For this review, use the dimensioned drawing (mm, ordinates from the lowest corner) and the shaded views. A direction names the side the tool comes from. Give positions to 0.01 mm unless a question says otherwise; leave off trailing zeros. Write each loop counter-clockwise with the first axis right and the second up, starting at its lowest first coordinate (ties: lowest second). Pieces come first, ordered by that corner, then holes. Notation, with made-up numbers: (44.25, 49.5) - (54.25, 49.5) arc R14 ccw to (54.25, 70.5) - close; hole circle Ø9 at (-13.75, 62.5). An arc over 180 degrees is marked (long way). One line per question, with ' | ' between items. Start each with the question number.
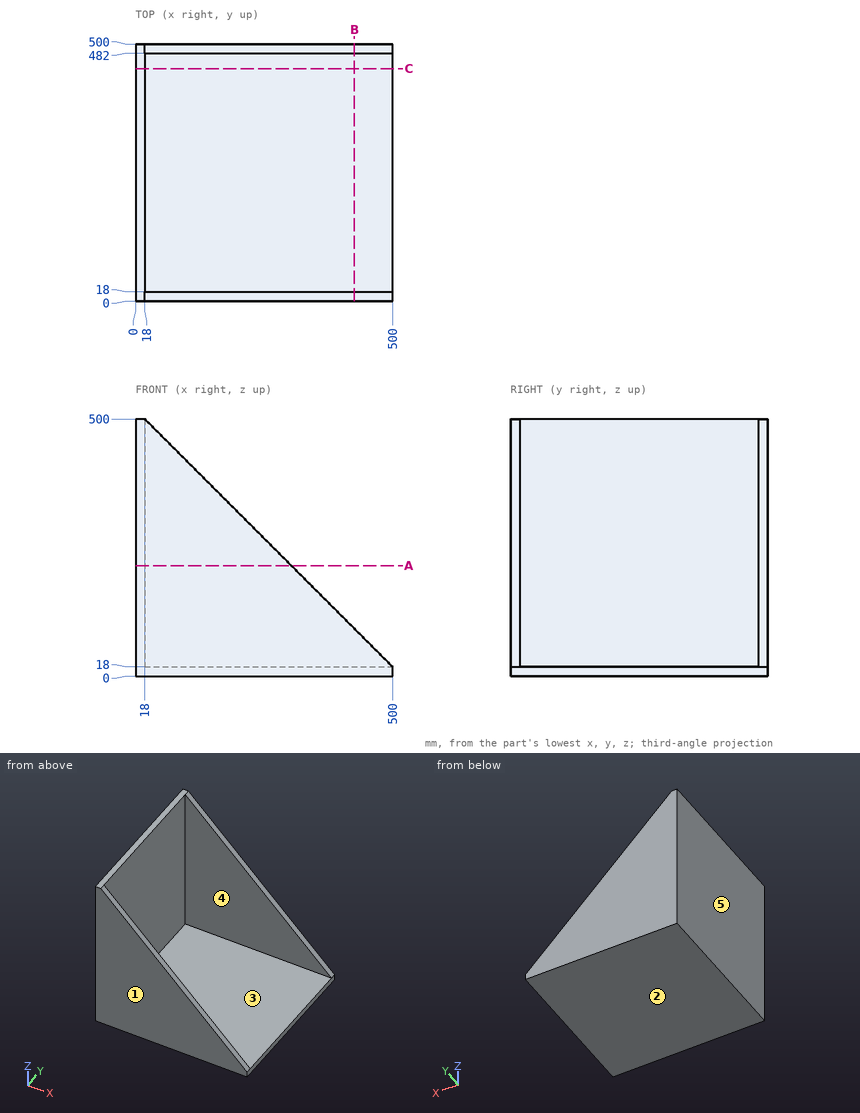
Item 1: Clearance check with a flat-ended pin moving along its axis: P1, Ø3, axis at x = 77.5, y = 74, coming from the +Z side. State where the tip first meets the part, or that it passes through.
Item 2: For probe 1 along Y at (x, z) = (302, 68); probe 2 along X at (y, z) = (246, 169.5), list the stretches that pass through material, from the lowest coordinate up.
Item 3: Machinability: for the marked faces 4 and 5, which of the approach directions +Z, -Z, +X, -X, +Y, -Y give a long, thin tool a straight path to every point of the face, cutting with its end or side? Answer none if there is none.
Item 4: Take a section at A-A (z = 214.5). Give the boundary of the cut face in (x, y), plus the area to 3 significant figures.
Item 5: Take a section at B-B (x = 426). Give the boundary of the cut face in (y, z), plus the area to 3 significant figures.
Item 6: The part is to be moulded in two halves that separate along Y. For the marked faces 1, 2 and 3, say which applies: +Y half, -Y half, draft (parallel to the pull), parting line (faces both ways), or undercut.
Item 7: Take a section at C-C (y = 452). Give the boundary of the cut face in (x, z).
Check sheet entries:
1) P1: stops at z = 18
2) probe 1: y = 0 to 18, 482 to 500 | probe 2: x = 0 to 18
3) face 4: +Z, +X | face 5: +Z, -Z, -X, +Y, -Y
4) outline: (0, 0) - (303.5, 0) - (303.5, 18) - (18, 18) - (18, 482) - (303.5, 482) - (303.5, 500) - (0, 500) - close | area: 19,300 mm^2
5) outline: (0, 0) - (500, 0) - (500, 92) - (482, 92) - (482, 18) - (18, 18) - (18, 92) - (0, 92) - close | area: 11,700 mm^2
6) face 1: -Y half | face 2: draft | face 3: undercut
7) outline: (0, 0) - (500, 0) - (500, 18) - (18, 18) - (18, 500) - (0, 500) - close
